Model file for the job. Use its own axes, mm. Give positions to 0.01 mm unless a question says otherwise; leave off trailing zeros. Write each loop counter-clockwise with the first axis right and the second up, starting at its lowest first coordinate (ties: lowest second). Pieces come first, ordered by that corner, then holes.
```python
from build123d import *

# Parameters (mm, degrees)
SKETCH1_R           = 4
SKETCH1_R_2         = 2.5
SKETCH1_R_3         = 3
BOSS_EXTRUDE1_DEPTH = 5
FILLET1_R           = 5


with BuildPart() as part:
    # Sketch1 → Boss-Extrude1 (new body)
    with BuildSketch(Plane.XY):
        Polygon((72, 0), (0, 0), (-30, -2.5), (-30, -47.5), (0, -50), (72, -50), (102, -47.5), (102, -2.5), align=None)
        with Locations((-22.5, -25)):
            Circle(SKETCH1_R, mode=Mode.SUBTRACT)
        with Locations((-7.5, -25)):
            Circle(SKETCH1_R, mode=Mode.SUBTRACT)
        with Locations((52, -43)):
            Circle(SKETCH1_R_2, mode=Mode.SUBTRACT)
        with Locations((52, -7)):
            Circle(SKETCH1_R_2, mode=Mode.SUBTRACT)
        with Locations((79.5, -25)):
            Circle(SKETCH1_R, mode=Mode.SUBTRACT)
        with Locations((94.5, -25)):
            Circle(SKETCH1_R, mode=Mode.SUBTRACT)
        with Locations((20, -25)):
            Circle(SKETCH1_R_2, mode=Mode.SUBTRACT)
        with Locations((52, -25)):
            Circle(SKETCH1_R_2, mode=Mode.SUBTRACT)
        with Locations((7, -25)):
            Circle(SKETCH1_R_3, mode=Mode.SUBTRACT)
        with Locations((65, -25)):
            Circle(SKETCH1_R_3, mode=Mode.SUBTRACT)
        with Locations((20, -7)):
            Circle(SKETCH1_R_2, mode=Mode.SUBTRACT)
        with Locations((20, -43)):
            Circle(SKETCH1_R_2, mode=Mode.SUBTRACT)
        with BuildLine():
            ThreePointArc((7, -40), (4, -43), (7, -46))
            ThreePointArc((7, -46), (10, -43), (7, -40))
        make_face(mode=Mode.SUBTRACT)
        with BuildLine():
            ThreePointArc((65, -46), (68, -43), (65, -40))
            ThreePointArc((65, -40), (62, -43), (65, -46))
        make_face(mode=Mode.SUBTRACT)
        with BuildLine():
            ThreePointArc((65, -10), (68, -7), (65, -4))
            ThreePointArc((65, -4), (62, -7), (65, -10))
        make_face(mode=Mode.SUBTRACT)
        with BuildLine():
            ThreePointArc((7, -10), (10, -7), (7, -4))
            ThreePointArc((7, -4), (4, -7), (7, -10))
        make_face(mode=Mode.SUBTRACT)
    extrude(amount=BOSS_EXTRUDE1_DEPTH)

    # Fillet1
    fillet1_edges = [part.edges().sort_by_distance(p)[0] for p in [
        (102, -2.5, 2.5),
        (102, -47.5, 2.5),
        (-30, -47.5, 2.5),
        (-30, -2.5, 2.5),
    ]]
    fillet(fillet1_edges, radius=FILLET1_R)


solid = part.part
```
1. Slice it at A-A, the plane x = 65. Write the cut outline in (y, z).
Calculated:
outline: (-50, 0) - (-46, 0) - (-46, 5) - (-50, 5) - close; (-40, 0) - (-28, 0) - (-28, 5) - (-40, 5) - close; (-22, 0) - (-10, 0) - (-10, 5) - (-22, 5) - close; (-4, 0) - (0, 0) - (0, 5) - (-4, 5) - close
2. Probe probe 1 along Y at (x, z) = (52, 1.95); probe 2 along Y at (x, z) = (65, 3.45); probe 3 along X at (y, z) = (-45, 1.5). List the from-to ranges inside material, lowest first.
Calculated:
probe 1: y = -50 to -45.5, -40.5 to -27.5, -22.5 to -9.5, -4.5 to 0
probe 2: y = -50 to -46, -40 to -28, -22 to -10, -4 to 0
probe 3: x = -29.54 to 4.76, 9.24 to 18.5, 21.5 to 50.5, 53.5 to 62.76, 67.24 to 101.54
3. Pull direction X, two halves, no side cores. Call faces 1 (the flat face through (35, -25, 5)), 2 (the cylindrical face through (-28.71, -46.25, 2.54)), 3 (the cylindrical face through (54.31, -43.96, 2.46)): +X half, -X half, draft (parallel to the pull), parting line (faces both ways), or undercut.
Calculated:
face 1: draft
face 2: -X half
face 3: undercut
4. Slice it at B-B, the plane z = 4.15. State how many separate pieces and enclosed holes the cut face has, and give its area (3 significant figures).
Calculated:
separate pieces: 1
enclosed holes: 16
area: 5,940 mm2
5. Pin check, flat tips, straight feed: P1, Ø1.5, axis at x = -16.5, z = 4, coming from the +Y side; P2, Ø3, axis at x = 20, y = -7, coming from the -Z side. Stop position of each tip, or through.
Calculated:
P1: stops at y = -1.31
P2: passes through
6. Slice it at C-C, the plane x = 79.5. Write the cut outline in (y, z) (3 decimals).
Calculated:
outline: (-49.375, 0) - (-29, 0) - (-29, 5) - (-49.375, 5) - close; (-21, 0) - (-0.625, 0) - (-0.625, 5) - (-21, 5) - close
